For this review, take the finished solid that the model builds, in its own axes (mm). Coordinates: 2 decimals unless noted, no trailing zeros. Loops run counter-clockwise (first coordinate to the right, second up) from the corner with the lowest first, then second, coordinate; pieces in that order, holes last. Notation, with made-up numbers: M 13,33.25 L 18,33.25 A34 cw 18,69.25 Z; hole C 8,84 d3. An arc over 180 degrees is marked long. Write each question's results on one line, items separated by ' | '. Start each with the question number.
Autodesk Inventor part; units mm, degrees
ref_plane "YZ Plane" through (0, 0, 0) normal (1, 0, 0) x (0, 1, 0)
ref_plane "XZ Plane" through (0, 0, 0) normal (0, 1, 0) x (-1, 0, 0)
ref_plane "XY Plane" through (0, 0, 0) normal (0, 0, 1) x (1, 0, 0)
sketch "Boceto1" plane through (0, 0, 0) normal (0, 1, 0) x (-1, 0, 0)
  circle A0 centre (0, 0) radius 4
  dimension "d0" = 8
extrude "Extrusión1" add sketch "Boceto1" along normal mid plane 80
sketch "Boceto2" plane through (0, 0, 0) normal (1, 0, 0) x (0, 1, 0)
  line L0 (44, 0) -> (44, -2)
  line L1 (44, 0) -> (40, 0)
  line L2 (40, -4) -> (40, 4)
  line L3 (40, 0) -> (40, -3.6)
  arc A0 (40.0881, -4.0105) -> (41.9882, -3.753) centre (41, -3.6) ccw
  arc A1 (40, -4) -> (40.0881, -4.0105) centre (40.5168, -0.0335) ccw
  arc A2 (41.9882, -3.753) -> (44, -2) centre (40.5168, -0.0335) ccw
  point P0 (0, 0)
  dimension "d4" = 4
  dimension "d6" = 2
  dimension "d8" = 0.4
revolve "Revolución1" add sketch "Boceto2" angle 360 about axis through (0, 44, 0) along (0, -1, 0)
mirror "Simetría1" about plane through (0, 0, 0) normal (0, 1, 0) of "Revolución1"
properties part number "Eje-Bisagra" material "Acero inoxidable"
Q1. The part is to be moulded in two halves that separate along Y. For faces 1 (the face through (0, -44, 0)), 2 (the face through (0, 44, 0)), 3 (the face through (0.867, -0.56, 3.905)), say which applies: pulls with the +Y half, pulls with the -Y half, needs draft (parallel to the pull), parting line crosses it, or undercut.
Q2. Take a section at A-A, the plane y = -21.5. Give the boundary of the cut face in (x, z).
Q3. To check wall thickness, follow line 1 along X through (y, z) = (7, -0.25); line 2 along Y through (x, z) = (-0.75, 4); line 3 along X through (y, z) = (-39, -2.25). State the ranges of each line that lie inside material, in increasing order.
Q4. Insertion check: P1, Ø3, axis at x = 0, y = 29, coming from the +Z side; P2, Ø4, axis at x = 2.5, z = -2.5, coming from the +Y side; P3, Ø2, axis at x = 3, y = -10, coming from the +Z side; P4, Ø4, axis at x = -0.5, y = 0.5, coming from the -Z side. Each pin has a flat end and moves straight along its axis. Give the tip position at first contact, or say it passes through.
Results:
1) face 1: pulls with the -Y half | face 2: pulls with the +Y half | face 3: undercut
2) outline: C 0,0 d8
3) line 1: -3.99 to 3.99 | line 2: -41.88 to -40.12, 40.12 to 41.88 | line 3: -3.31 to 3.31
4) P1: z = 4 | P2: y = 44 | P3: z = 3.46 | P4: z = -4
